Check sheet for the drawn part. Datum: minimum x, y, z corner. Units: mm. A direction names the side the tool comes from. Round coordinates to 2 decimals unless told otherwise and drop trailing zeros. Write each loop counter-clockwise with the first axis right and the second up, starting at its lowest first coordinate (ties: lowest second). Pieces come first, ordered by that corner, then holes. Notation, with made-up numbers: M 67,86.25 L 94,86.25 A14 cw 94,111.25 Z; hole C -9.75,15 d3. An arc over 180 degrees is marked long. Put each result on its own line as item: value.
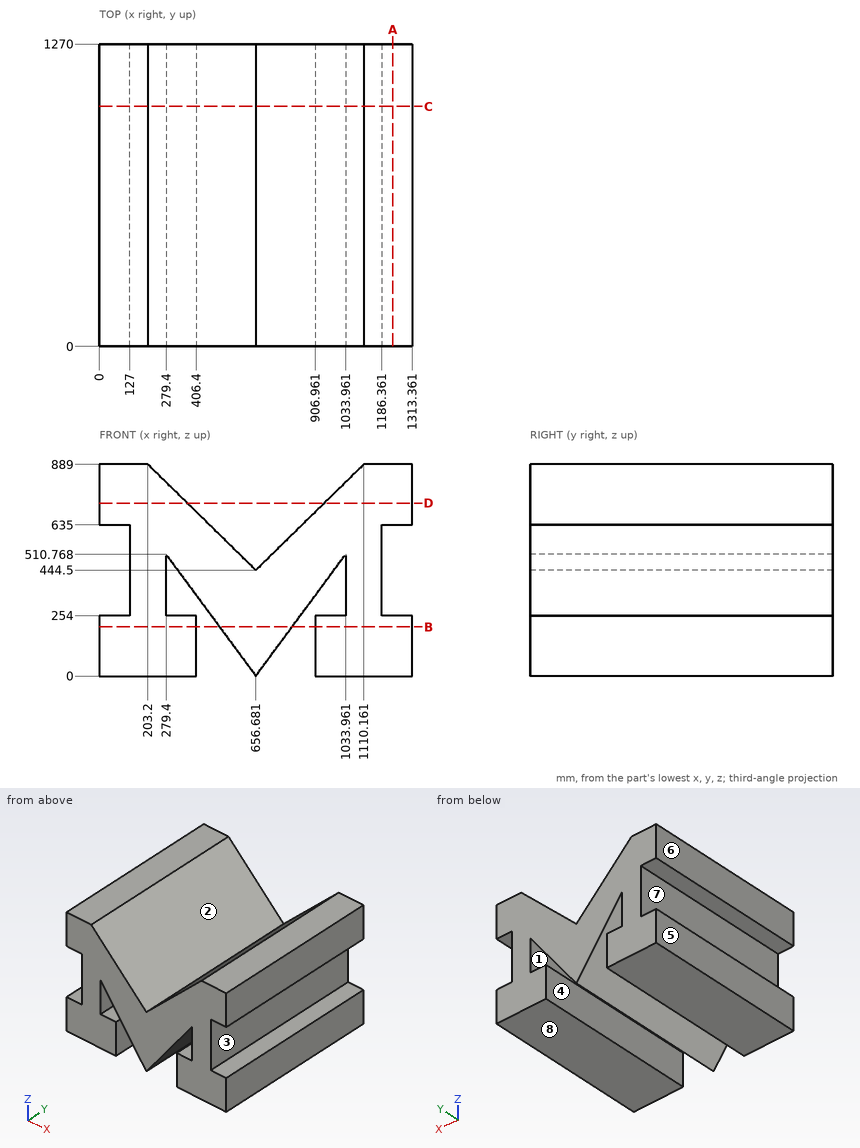
1. Scan lines: probe 1 along Z at (x, y) = (81, 104); probe 2 along X at (y, z) = (1214, 120); probe 3 along X at (y, z) = (384, 252.5). Record each from-to range of solid material in increasing order.
Computed values:
probe 1: z = 0 to 254, 635 to 889
probe 2: x = 0 to 406.4, 568.04 to 745.32, 906.96 to 1313.36
probe 3: x = 0 to 406.4, 470.17 to 843.19, 906.96 to 1313.36
2. Depth check by flat-ended pin: pin 1 Ø3 at (x, y) = (266.5, 895) entering from +Z (1 decimal); pin 2 Ø1 at (y, z) = (372.5, 622) entering from -X; pin 3 Ø12 at (x, y) = (289.5, 194.5) entering from +Z. Enter the tip coordinate at first touch or a pass-through.
Computed values:
pin 1: stops at z = 828.4
pin 2: stops at x = 127
pin 3: stops at z = 810.29
3. Cross-section at A-A (x = 1232). Enter the section's corners in (y, z), then the cut area to 3 significant figures.
Computed values:
outline: M 0,0 L 1270,0 L 1270,254 L 0,254 Z; M 0,635 L 1270,635 L 1270,889 L 0,889 Z
area: 645,000 mm2
4. Cross-section at B-B (z = 206.5). Enter the section's corners in (x, y).
Computed values:
outline: M 0,0 L 406.4,0 L 406.4,1270 L 0,1270 Z; M 504.15,0 L 809.21,0 L 809.21,1270 L 504.15,1270 Z; M 906.96,0 L 1313.36,0 L 1313.36,1270 L 906.96,1270 Z
5. Access from +Z, -Z, +X, -X, +Y, -Y to the whole of each face (thin tool, end or side, straight path). Record for the marked faces 1, 2, 3, 4 and 5.
Computed values:
face 1: +Y, -Y
face 2: +Z, +Y, -Y
face 3: +X, +Y, -Y
face 4: -Z, +Y, -Y
face 5: +Z, -Z, -X, +Y, -Y
6. Cross-section at C-C (y = 1008). Enter the section's corners in (x, z).
Computed values:
outline: M 0,0 L 406.4,0 L 406.4,254 L 279.4,254 L 279.4,510.77 L 656.68,0 L 1033.96,510.77 L 1033.96,254 L 906.96,254 L 906.96,0 L 1313.36,0 L 1313.36,254 L 1186.36,254 L 1186.36,635 L 1313.36,635 L 1313.36,889 L 1110.16,889 L 656.68,444.5 L 203.2,889 L 0,889 L 0,635 L 127,635 L 127,254 L 0,254 Z
7. Release check for a two-part mould opening along Z. For the marked faces 6, 7 and 8 record: +Z half, -Z half, draft (parallel to the pull), parting line (faces both ways), or undercut.
Computed values:
face 6: draft
face 7: undercut
face 8: -Z half
8. Cross-section at D-D (z = 726). Enter the section's corners in (x, y).
Computed values:
outline: M 0,0 L 369.49,0 L 369.49,1270 L 0,1270 Z; M 943.87,0 L 1313.36,0 L 1313.36,1270 L 943.87,1270 Z
